Read the model definition and answer for the solid it produces. Units are mm, in the model's axes. A direction names the side the tool comes from. Coordinates: 2 decimals unless noted, no trailing zeros. Order: outer loops, then holes, each group sorted by start corner. A loop starts at its lowest first (then second) coordinate and runs counter-clockwise, first axis right, second up.
```python
from build123d import *

# Parameters (mm, degrees)
SKETCH1_R           = 6
SKETCH1_R_2         = 3
BOSS_EXTRUDE1_DEPTH = 4.2
SKETCH2_R           = 12.7
SKETCH2_R_2         = 3
BOSS_EXTRUDE2_DEPTH = 5
SKETCH3_R           = 1.4
CUT_EXTRUDE1_DEPTH  = 13.7
SKETCH4_R           = 1.4
CUT_EXTRUDE2_DEPTH  = 5


with BuildPart() as part:
    # Sketch1 → Boss-Extrude1 (new body)
    with BuildSketch(Plane.XY):
        Circle(SKETCH1_R)
        Circle(SKETCH1_R_2, mode=Mode.SUBTRACT)
    extrude(amount=BOSS_EXTRUDE1_DEPTH)

    # Sketch2 → Boss-Extrude2 (add)
    with BuildSketch(Plane.XY.offset(4.2)):
        Circle(SKETCH2_R)
        Circle(SKETCH2_R_2, mode=Mode.SUBTRACT)
    extrude(amount=BOSS_EXTRUDE2_DEPTH)

    # Sketch3 → Cut-Extrude1 (cut, through all)
    with BuildSketch(Plane(origin=(0, 0, 0), x_dir=(1, 0, 0), z_dir=(0, 1, 0))):
        with Locations((0, -2.1)):
            Circle(SKETCH3_R)
    extrude(amount=-CUT_EXTRUDE1_DEPTH, mode=Mode.SUBTRACT)

    # Sketch4 → Cut-Extrude2 (cut)
    with BuildSketch(Plane.XY.offset(9.2)):
        with Locations((0, 9.5)):
            Circle(SKETCH4_R)
        with Locations((8.227241336, 4.75)):
            Circle(SKETCH4_R)
        with Locations((8.227241336, -4.75)):
            Circle(SKETCH4_R)
        with Locations((0, -9.5)):
            Circle(SKETCH4_R)
        with Locations((-8.227241336, -4.75)):
            Circle(SKETCH4_R)
        with Locations((-8.227241336, 4.75)):
            Circle(SKETCH4_R)
    extrude(amount=-CUT_EXTRUDE2_DEPTH, mode=Mode.SUBTRACT)


solid = part.part
```
1) Determine the mould class of faces 3 (the flat face through (3, -3, 9.2)), 4 (the cylindrical face through (-2.75, -12.4, 6.66)), 5 (the cylindrical face through (-0.303, -4.305, 3.467)) for opening direction Z: pulls with the +Z half, pulls with the -Z half, needs draft (parallel to the pull), parting line crosses it, or undercut.
A:
face 3: pulls with the +Z half
face 4: needs draft
face 5: undercut
2) Which of the six approach directions +Z, -Z, +X, -X, +Y, -Y give full straight-line access (tool end or side, diameter ignored) to faces 1 (the flat face through (5.5, 3, 4.2)), 2 (the cylindrical face through (9.563, 5.171, 6.735))?
A:
face 1: -Z
face 2: +Z, -Z
3) Flat-ended cylindrical pins translate along their axes: pin 1 Ø3 at (x, z) = (0, 2.1) entering from +Y; pin 2 Ø3 at (x, z) = (0, 2.5) entering from -Y; pin 3 Ø4.5 at (x, y) = (8.23, -4.75) entering from -Z. Find the tip coordinate at first contact, or state that the pin passes through.
A:
pin 1: stops at y = 6
pin 2: stops at y = -6
pin 3: stops at z = 4.2
4) Straight lines are drawn through the part: line 1 (Y direction, x = 0, z = 5.6); line 2 (Z direction, x = 0, y = -5.2); line 3 (Y direction, x = -9.5, z = 7.5). For each, find the intervals that lie inside material, in ascending order.
A:
line 1: y = -12.7 to -10.9, -8.1 to -3, 3 to 8.1, 10.9 to 12.7
line 2: z = 0 to 0.7, 3.5 to 9.2
line 3: y = -8.43 to -5.33, -4.17 to 4.17, 5.33 to 8.43
5) A cutting plane is placed at D-D, the plane y = -4.75. Determine the outline of the cut face in (x, z), and give its area (3 significant figures).
A:
outline: (-11.78, 4.2) - (-9.63, 4.2) - (-9.63, 9.2) - (-11.78, 9.2) - close; (-6.83, 4.2) - (-3.67, 4.2) - (-3.67, 0) - (3.67, 0) - (3.67, 4.2) - (6.83, 4.2) - (6.83, 9.2) - (-6.83, 9.2) - close; (9.63, 4.2) - (11.78, 4.2) - (11.78, 9.2) - (9.63, 9.2) - close; hole circle Ø2.8 at (0, 2.1)
area: 114 mm2
6) A cutting plane is placed at B-B, the plane y = 0. Determine the outline of the cut face in (x, z).
A:
outline: (-12.7, 4.2) - (-6, 4.2) - (-6, 0) - (-3, 0) - (-3, 9.2) - (-12.7, 9.2) - close; (3, 0) - (6, 0) - (6, 4.2) - (12.7, 4.2) - (12.7, 9.2) - (3, 9.2) - close
7) A cutting plane is placed at C-C, the plane x = -0.25. Determine the outline of the cut face in (y, z), and give its area (3 significant figures).
A:
outline: (-12.7, 4.2) - (-10.88, 4.2) - (-10.88, 9.2) - (-12.7, 9.2) - close; (-8.12, 4.2) - (-5.99, 4.2) - (-5.99, 3.48) - (-2.99, 3.48) - (-2.99, 9.2) - (-8.12, 9.2) - close; (-5.99, 0) - (-2.99, 0) - (-2.99, 0.72) - (-5.99, 0.72) - close; (2.99, 0) - (5.99, 0) - (5.99, 4.2) - (8.12, 4.2) - (8.12, 9.2) - (2.99, 9.2) - close; (10.88, 4.2) - (12.7, 4.2) - (12.7, 9.2) - (10.88, 9.2) - close
area: 86.5 mm2
8) A cutting plane is placed at A-A, the plane z = 5. Determine the outline of the cut face in (x, y).
A:
outline: circle Ø25.4 at (0, 0); hole circle Ø2.8 at (-8.23, -4.75); hole circle Ø2.8 at (-8.23, 4.75); hole circle Ø6 at (0, 0); hole circle Ø2.8 at (0, -9.5); hole circle Ø2.8 at (0, 9.5); hole circle Ø2.8 at (8.23, -4.75); hole circle Ø2.8 at (8.23, 4.75)
